Can you work these out from the drawing? Everything is in mm from the part's minimum corner. A direction names the side the tool comes from. Coordinates: 2 decimals unless noted, no trailing zeros. Order: outer loops, then holes, each group sorted by start corner. A loop starts at its lowest first (then second) coordinate and runs counter-clockwise, first axis right, second up. Notation, with made-up numbers: (24.5, 88.25) -> (29.5, 88.25) arc R16 cw to (29.5, 111.25) -> close; hole circle Ø8 at (38, -30). An arc over 180 degrees is marked (long way). Put each result on its own line as item: value. Start each with the question number.
Q1. If we section it at C-C (z = 6.5): Please give me the cut outline in (x, y).
Q2. Please list where these lines run through material, in increasing order: line 1 along X through (y, z) = (15, 4.5); line 2 along X through (y, z) = (65, 12.25).
Q3. Will these pins go through, and if not, where does the flat tip stop? pin 1 (1.2 mm diameter, centred on y = 62, z = 12, fed in from -X); pin 2 (4.5 mm diameter, centred on x = 7.15, y = 64.85, fed in from +Z); pin 3 (1.8 mm diameter, centred on y = 64.5, z = 8.5, fed in from +X) (3 decimals); pin 4 (8 mm diameter, centred on x = 40, y = 59, fed in from +Z).
Q4. If we section it at A-A (x = 50.5): Please give me the cut outline in (y, z).
Q5. We'd pull the mould along Y, two halves only. Please class the marked faces 3, 4 and 5: +Y half, -Y half, draft (parallel to the pull), parting line (faces both ways), or undercut.
Q6. For the marked faces 1 and 2, which set-ups out of +Z, -Z, +X, -X, +Y, -Y let a thin tool reach every point of the face, with its end or its side?
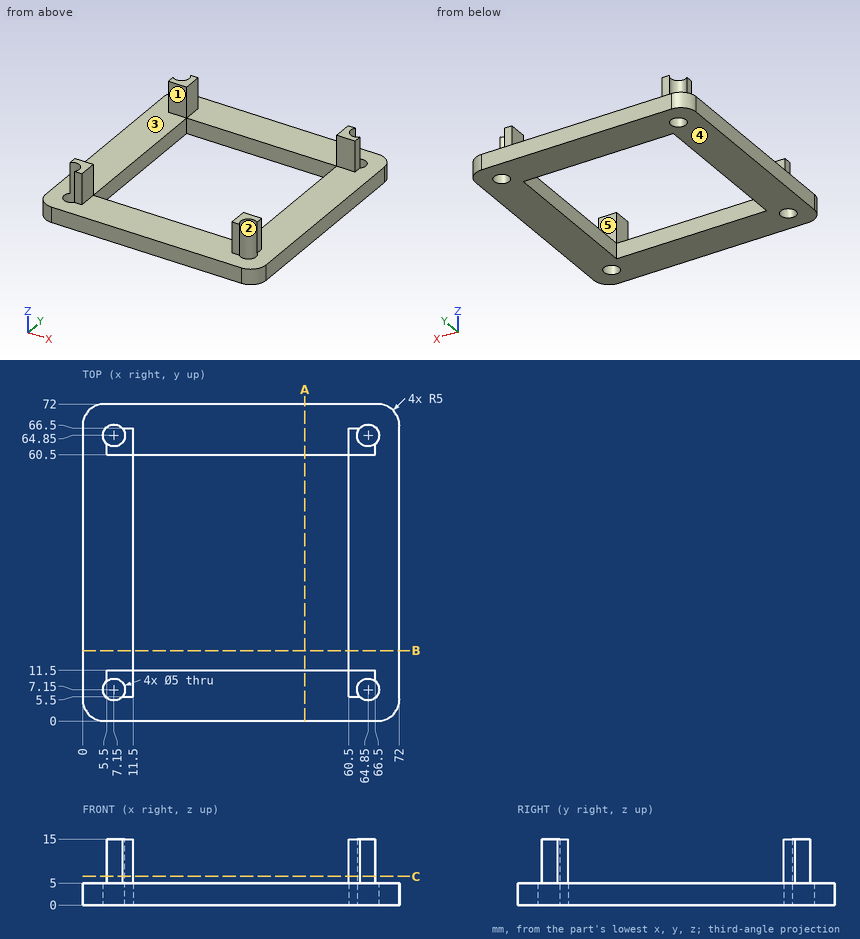
The answers:
1. outline: (5.5, 9.03) arc R2.5 cw to (9.03, 5.5) -> (11.5, 5.5) -> (11.5, 11.5) -> (5.5, 11.5) -> close; (5.5, 60.5) -> (11.5, 60.5) -> (11.5, 66.5) -> (9.03, 66.5) arc R2.5 cw to (5.5, 62.97) -> close; (60.5, 5.5) -> (62.97, 5.5) arc R2.5 cw to (66.5, 9.03) -> (66.5, 11.5) -> (60.5, 11.5) -> close; (60.5, 60.5) -> (66.5, 60.5) -> (66.5, 62.97) arc R2.5 cw to (62.97, 66.5) -> (60.5, 66.5) -> close
2. line 1: 0 to 11.5, 60.5 to 72
2. line 2: 9.65 to 11.5, 60.5 to 62.35
3. pin 1: x = 5.5
3. pin 2: through
3. pin 3: x = 62.685
3. pin 4: z = 5
4. outline: (0, 0) -> (11.5, 0) -> (11.5, 5) -> (0, 5) -> close; (60.5, 0) -> (72, 0) -> (72, 5) -> (60.5, 5) -> close
5. face 3: undercut
5. face 4: draft
5. face 5: undercut
6. face 1: +Z, +X, -X
6. face 2: +Z, -Z
